from build123d import *

# Parameters (mm, degrees)
ESBO_O1_W                = 30
ESBO_O1_H                = 60
RESSALTO_EXTRUS_O1_DEPTH = 20
CORTE_EXTRUS_O1_DEPTH    = 17
ESBO_O7_R                = 3
ESBO_O7_R_2              = 5
CORTE_EXTRUS_O2_DEPTH    = 17
ESBO_O9_R                = 3
CORTE_EXTRUS_O4_DEPTH    = 71


with BuildPart() as part:
    # Esboço1 → Ressalto-extrusão1 (new body)
    with BuildSketch(Plane.XY):
        with Locations((15, 30)):
            Rectangle(ESBO_O1_W, ESBO_O1_H)
    extrude(amount=RESSALTO_EXTRUS_O1_DEPTH)

    # Esboço6 → Corte-extrusão1 (cut)
    with BuildSketch(Plane.XY.offset(20)):
        Polygon((28, 58), (15, 58), (2, 58), (2, 2), (15, 2), (28, 2), align=None)
    extrude(amount=-CORTE_EXTRUS_O1_DEPTH, mode=Mode.SUBTRACT)

    # Esboço7 → Corte-extrusão2 (cut)
    with BuildSketch(Plane.XY.offset(3)):
        with Locations((15, 10)):
            Circle(ESBO_O7_R)
        with Locations((15, 50)):
            Circle(ESBO_O7_R)
        with Locations((15, 30)):
            Circle(ESBO_O7_R_2)
    extrude(amount=-CORTE_EXTRUS_O2_DEPTH, mode=Mode.SUBTRACT)

    # Esboço9 → Corte-extrusão4 (cut, through all)
    with BuildSketch(Plane(origin=(30, 0, 0), x_dir=(0, 0, -1), z_dir=(1, 0, 0))):
        with Locations((-13, 50)):
            Circle(ESBO_O9_R)
        with Locations((-13, 10)):
            Circle(ESBO_O9_R)
    extrude(amount=-CORTE_EXTRUS_O4_DEPTH, mode=Mode.SUBTRACT)


solid = part.part
The model under review builds one solid part; all positions refer to its coordinate system, in mm. A direction names the side the tool comes from. Round coordinates to 2 decimals unless told otherwise and drop trailing zeros. Loops run counter-clockwise (first coordinate to the right, second up) from the corner with the lowest first, then second, coordinate; pieces in that order, holes last. Notation, with made-up numbers: M 15,61 L 37,61 A23 ccw 37,97 Z; hole C 65,88.25 d3. An arc over 180 degrees is marked long. Answer as a JSON object with one key per item and string values.
Item 1: For line 1 along Y through (x, z) = (15, 2); line 2 along Y through (x, z) = (1.4, 13); line 3 along Y through (x, z) = (15.25, 4.5), list the stretches that pass through material, from the lowest coordinate up.
Check sheet entries:
{"line 1": "0 to 7, 13 to 25, 35 to 47, 53 to 60", "line 2": "0 to 7, 13 to 47, 53 to 60", "line 3": "0 to 2, 58 to 60"}
Item 2: We need section B-B, the plane y = 30. State the section outline as (x, z) points.
Check sheet entries:
{"outline": "M 0,0 L 10,0 L 10,3 L 2,3 L 2,20 L 0,20 Z; M 20,0 L 30,0 L 30,20 L 28,20 L 28,3 L 20,3 Z"}
Item 3: The part is to be moulded in two halves that separate along X. For faces 3 (the face through (15, 0, 10)), 4 (the face through (19.619, 28.085, 1.521)), 5 (the face through (30, 30, 10)), say which applies: +X half, -X half, draft (parallel to the pull), parting line (faces both ways), or undercut.
Check sheet entries:
{"face 3": "draft", "face 4": "undercut", "face 5": "+X half"}
Item 4: We need section A-A, the plane y = 10. State the section outline as (x, z) points.
Check sheet entries:
{"outline": "M 0,0 L 12,0 L 12,3 L 2,3 L 2,10 L 0,10 Z; M 0,16 L 2,16 L 2,20 L 0,20 Z; M 18,0 L 30,0 L 30,10 L 28,10 L 28,3 L 18,3 Z; M 28,16 L 30,16 L 30,20 L 28,20 Z"}
Item 5: Tool access review of faces 1 (the face through (1, 8.2, 15.4)), 2 (the face through (15, 58, 12)): name each direction out of +Z, -Z, +X, -X, +Y, -Y from which nothing blocks a thin tool from reaching the whole face with its end or side.
Check sheet entries:
{"face 1": "+X, -X", "face 2": "+Z"}
Item 6: We need section D-D, the plane z = 13. State the section outline as (x, y) points, and give its area (3 significant figures).
Check sheet entries:
{"outline": "M 0,0 L 30,0 L 30,7 L 28,7 L 28,2 L 2,2 L 2,7 L 0,7 Z; M 0,13 L 2,13 L 2,47 L 0,47 Z; M 0,53 L 2,53 L 2,58 L 28,58 L 28,53 L 30,53 L 30,60 L 0,60 Z; M 28,13 L 30,13 L 30,47 L 28,47 Z", "area": "296 mm2"}
Item 7: We need section C-C, the plane x = 15. State the section outline as (y, z) points, and give its area (3 significant figures).
Check sheet entries:
{"outline": "M 0,0 L 7,0 L 7,3 L 2,3 L 2,20 L 0,20 Z; M 13,0 L 25,0 L 25,3 L 13,3 Z; M 35,0 L 47,0 L 47,3 L 35,3 Z; M 53,0 L 60,0 L 60,20 L 58,20 L 58,3 L 53,3 Z", "area": "182 mm2"}
Item 8: Clearance check with a flat-ended pin moving along its axis: P1, Ø12, axis at x = 14, y = 13.5, coming from the +Z side. State where the tip first meets the part, or that it passes through.
Check sheet entries:
{"P1": "z = 3"}
